```python
from build123d import *

# Parameters (mm, degrees)
F0_W     = 125
F0_H     = 40
F1_DEPTH = 3
F2_W     = 119
F2_H     = 34
F3_DEPTH = 3
F4_W     = 55
F4_H     = 14.9112120271
F5_DEPTH = 34
F6_R     = 5


with BuildPart() as f1:
    # F0 (on Front) → F1 (new body)
    with BuildSketch(Plane.XZ):
        Rectangle(F0_W, F0_H)
        with BuildLine():
            ThreePointArc((62.5, -20), (82.5, 0), (62.5, 20))
            Line((62.5, 20), (62.5, -20))
        make_face()
        with BuildLine():
            Line((-62.5, -20), (-62.5, 20))
            ThreePointArc((-62.5, 20), (-82.5, 0), (-62.5, -20))
        make_face()
    extrude(amount=F1_DEPTH)

    # F2 (on face) → F3 (join)
    with BuildSketch(Plane.XZ.offset(3)):
        Rectangle(F2_W, F2_H)
        with BuildLine():
            ThreePointArc((59.5, -17), (76.5, 0), (59.5, 17))
            Line((59.5, 17), (59.5, -17))
        make_face()
        with BuildLine():
            Line((-59.5, -17), (-59.5, 17))
            ThreePointArc((-59.5, 17), (-76.5, 0), (-59.5, -17))
        make_face()
    extrude(amount=F3_DEPTH)

    # F4 (on face) → F5 (join)
    with BuildSketch(Plane.XY.offset(17)):
        with Locations((0, -9.8109263927)):
            Rectangle(F4_W, F4_H)
        with BuildLine():
            ThreePointArc((-39.5, -6), (-34.1717325339, -12.3487294988), (-27.5, -17.2665324062))
            Line((-27.5, -17.2665324062), (-27.5, -2.3553203791))
            Line((-27.5, -2.3553203791), (-39.5, -6))
        make_face()
        with BuildLine():
            Line((27.5, -2.3553203791), (27.5, -17.2665324062))
            ThreePointArc((27.5, -17.2665324062), (34.1717325339, -12.3487294988), (39.5, -6))
            Line((39.5, -6), (27.5, -2.3553203791))
        make_face()
    extrude(amount=-F5_DEPTH)

    # F6
    f6_edges = [f1.edges().sort_by_distance(p)[0] for p in [
        (-27.5, -17.266532, 0),
        (27.5, -17.266532, 0),
        (39.5, -6, 0),
        (-39.5, -6, 0),
    ]]
    fillet(f6_edges, radius=F6_R)


solid = f1.part
```
Verification items for the finished model (mm, model axes). A direction names the side the tool comes from. Round coordinates to 2 decimals unless told otherwise and drop trailing zeros. Order: outer loops, then holes, each group sorted by start corner. A loop starts at its lowest first (then second) coordinate and runs counter-clockwise, first axis right, second up.
1) Tool access check on faces 1 (the flat face through (0, -3, -18)), 2 (the flat face through (-60, -6, 0)), 3 (the flat face through (-1, -8, 17)), 4 (the flat face through (-1, -8, -17)), 5 (the flat face through (59, -6, 0)). Record the directions out of +Z, -Z, +X, -X, +Y, -Y that give a thin tool (end or side, any length) a straight path to the whole face; none if there is none.
Geometry says:
face 1: -Y
face 2: +Z, -Z, -X, -Y
face 3: +Z, +X, -X, -Y
face 4: -Z, +X, -X, -Y
face 5: +Z, -Z, +X, -Y
2) Cross-section at A-A, the plane z = 0. Record the cut outline in (x, y), plus the area to 3 significant figures.
Geometry says:
outline: (-82.5, -3) - (-76.5, -3) - (-76.5, -6) - (-42.09, -6) arc R5 cw to (-38.1, -7.98) arc R35 ccw to (-28.78, -16.51) arc R5 ccw to (-26.12, -17.27) - (26.12, -17.27) arc R5 ccw to (28.78, -16.51) arc R35 ccw to (38.1, -7.98) arc R5 cw to (42.09, -6) - (76.5, -6) - (76.5, -3) - (82.5, -3) - (82.5, 0) - (-82.5, 0) - close
area: 1,730 mm2
3) Material ranges on line 1 (Y direction, x = 8, z = 18); line 2 (X direction, y = -8, z = -16.5); line 3 (Y direction, x = 68, z = -3.5), recorded low to high.
Geometry says:
line 1: y = -3 to 0
line 2: x = -38.09 to 38.09
line 3: y = -6 to 0
4) Cross-section at B-B, the plane x = -10. Record the cut outline in (y, z), plus the area to 3 significant figures.
Geometry says:
outline: (-17.27, -17) - (-3, -17) - (-3, -20) - (0, -20) - (0, 20) - (-3, 20) - (-3, 17) - (-17.27, 17) - close
area: 605 mm2
5) Cross-section at D-D, the plane x = 47. Record the cut outline in (y, z).
Geometry says:
outline: (-6, -17) - (-3, -17) - (-3, -20) - (0, -20) - (0, 20) - (-3, 20) - (-3, 17) - (-6, 17) - close
6) Depth check by flat-ended pin: pin 1 (2 mm diameter, centred on x = -30.5, y = -14, fed in from +Z); pin 2 (1.5 mm diameter, centred on x = 33, z = 4.5, fed in from +Y); pin 3 (4 mm diameter, centred on x = -52.5, z = -13.5, fed in from -Y); pin 4 (1.5 mm diameter, centred on y = -2, z = 5.5, fed in from +X). Enter the tip coordinate at first touch or a pass-through.
Geometry says:
pin 1: stops at z = 17
pin 2: stops at y = 0
pin 3: stops at y = -6
pin 4: stops at x = 81.93
7) Cross-section at C-C, the plane y = -4.5. Record the cut outline in (x, z).
Geometry says:
outline: (-59.5, -17) - (59.5, -17) arc R17 ccw to (59.5, 17) - (-59.5, 17) arc R17 ccw to start
